from build123d import *

# Parameters (mm, degrees)
F1_DEPTH = 9
F2_R     = 18.012252
F3_DEPTH = 25


with BuildPart() as f1:
    # F0 (on Right) → F1 (new body)
    with BuildSketch(Plane.YZ):
        Polygon((10, 40), (10, 49), (-10, 49), (-10, 40), (-35, 40), (-35, 10), (-26, 10), (-26, -10), (-35, -10), (-35, -40), (-10, -40), (-10, -49), (10, -49), (10, -40), (35, -40), (35, 40), align=None)
    extrude(amount=F1_DEPTH)

    # F2 (on face) → F3 (join)
    with BuildSketch(Plane.YZ.offset(9)):
        Circle(F2_R)
    extrude(amount=F3_DEPTH)


solid = f1.part
The listing builds one solid part. Answer for the finished solid, in the listing's coordinates (mm). A direction names the side the tool comes from. Give positions to 0.01 mm unless a question says otherwise; leave off trailing zeros. Loops run counter-clockwise (first coordinate to the right, second up) from the corner with the lowest first, then second, coordinate; pieces in that order, holes last. Notation, with made-up numbers: (-32, 30.5) - (27, 30.5) arc R25 ccw to (27, 55.5) - close; hole circle Ø3 at (14.25, 48.25). An arc over 180 degrees is marked (long way). Write each question's results on one line, items separated by ' | '.
1. Find section D-D, the plane y = 0. Write down the section's boundary in (x, z), then the cut area to 3 significant figures.
Resolved:
outline: (0, -49) - (9, -49) - (9, -18.01) - (34, -18.01) - (34, 18.01) - (9, 18.01) - (9, 49) - (0, 49) - close | area: 1,780 mm^2
2. Find section C-C, the plane x = 6. Write down the section's boundary in (y, z), then the cut area to 3 significant figures.
Resolved:
outline: (-35, -40) - (-10, -40) - (-10, -49) - (10, -49) - (10, -40) - (35, -40) - (35, 40) - (10, 40) - (10, 49) - (-10, 49) - (-10, 40) - (-35, 40) - (-35, 10) - (-26, 10) - (-26, -10) - (-35, -10) - close | area: 5,780 mm^2
3. Which of the six approach directions +Z, -Z, +X, -X, +Y, -Y give full straight-line access (tool end or side, diameter ignored) to faces 1 (the face through (4, -26, 0)), 2 (the face through (4, 10, 44)), 3 (the face through (4, 10, -45)), 4 (the face through (21.325, -14.294, -10.96)), 5 (the face through (4, -10, 45))?
Resolved:
face 1: +X, -X, -Y | face 2: +Z, +X, -X, +Y | face 3: -Z, +X, -X, +Y | face 4: +X | face 5: +Z, +X, -X, -Y
4. Find section B-B, the plane z = 0. Write down the section's boundary in (x, y), then the cut area to 3 significant figures.
Resolved:
outline: (0, -26) - (9, -26) - (9, -18.01) - (34, -18.01) - (34, 18.01) - (9, 18.01) - (9, 35) - (0, 35) - close | area: 1,450 mm^2
5. Consider probe 1 along X at (y, z) = (24, 15.5); probe 2 along Z at (x, y) = (2.5, -23.5); probe 3 along Z at (x, y) = (18.5, 0.5). Determine where each line is inside the solid, lowest interval first. Write a range as from..to.
Resolved:
probe 1: x = 0..9 | probe 2: z = -40..40 | probe 3: z = -18.01..18.01
6. Flat-ended cylindrical pins translate along their axes: P1, Ø2.5, axis at x = 3, z = -46, coming from the +Y side; P2, Ø7, axis at x = 6.5, z = -46.5, coming from the -Y side; P3, Ø8, axis at y = -11.5, z = 22.5, coming from the -X side; P4, Ø4.5, axis at x = 6, z = -3, coming from the -Y side. Find the tip coordinate at first contact, or state that the pin passes through.
Resolved:
P1: stops at y = 10 | P2: stops at y = -10 | P3: stops at x = 0 | P4: stops at y = -26
7. For a pull along Z with two mould halves and no side action, classify faces 6 (the face through (4, -30, -10)), 7 (the face through (4, 22, -40)), 8 (the face through (4, 23, 40)) as +Z half, -Z half, draft (parallel to the pull), parting line (faces both ways), or undercut.
Resolved:
face 6: undercut | face 7: -Z half | face 8: +Z half
8. Find section A-A, the plane y = -27.5. Write down the section's boundary in (x, z).
Resolved:
outline: (0, -40) - (9, -40) - (9, -10) - (0, -10) - close; (0, 10) - (9, 10) - (9, 40) - (0, 40) - close
